For this review, take the finished solid that the model builds, in its own axes (mm). Round coordinates to 2 decimals unless told otherwise and drop trailing zeros. Order: outer loops, then holes, each group sorted by start corner. A loop starts at its lowest first (then second) coordinate and runs counter-clockwise, first axis right, second up. Notation, with made-up numbers: M 29.5,50.25 L 73.5,50.25 A5 ccw 73.5,56.25 Z; hole C 18,-35 d4. An arc over 180 degrees is marked long. Answer in a Markdown table with one row per item. Add a question column.
```python
from build123d import *

# Parameters (mm, degrees)
CYLINDER220_R     = 1.5
CYLINDER220_DEPTH = 10
CYLINDER093_R     = 4.1
CYLINDER093_DEPTH = 6.6


with BuildPart() as cylinder220:
    # Cylinder220 → Cylinder220 (new body)
    with BuildSketch(Plane.XY.offset(-1.9)):
        Circle(CYLINDER220_R)
    extrude(amount=CYLINDER220_DEPTH)


with BuildPart() as cut006:
    # Cylinder093 → Cylinder093 (new body)
    with BuildSketch(Plane.XY):
        Circle(CYLINDER093_R)
    extrude(amount=CYLINDER093_DEPTH)

    # Cut006: cut Cylinder220
    add(cylinder220.part, mode=Mode.SUBTRACT)


with BuildPart() as cut006_1:
    # Cut006 placement: moved
    add(cut006.part.moved(Location((76.8, 197.2, 52.1))))


solid = cut006_1.part
```
1. Consider section A-A on x = 76.8. Write out the cut boundary in (y, z), plus the area to 3 significant figures.
2. Clearance check with a flat-ended pin moving along its axis: pin 1 Ø1.5 at (y, z) = (198.5, 55.5) entering from -X. State where the tip first meets the part, or that it passes through.
3. Consider section D-D on x = 74.5. Write out the cut boundary in (y, z), plus the area to 3 significant figures.
4. The part is to be moulded in two halves that separate along Y. For faces 1 (the flat face through (77, 195, 52.1)), 2 (the cylindrical face through (78.69, 193.56, 55.35)), 3 (the cylindrical face through (76.475, 195.736, 55.354)), say which applies: pulls with the +Y half, pulls with the -Y half, needs draft (parallel to the pull), parting line crosses it, or undercut.
5. To check wall thickness, follow probe 1 along Y at (x, z) = (76.8, 55.5); probe 2 along X at (y, z) = (197.75, 56.75); probe 3 along X at (y, z) = (197, 54.25). State the ranges of each line that lie inside material, in increasing order. Write a range as [from, to].
6. Consider section B-B on y = 197.2. Write out the cut boundary in (x, z), plus the area to 3 significant figures.
7. Consider section C-C on z = 55. Write out the cut boundary in (x, y), plus the area to 3 significant figures.
Solved:
| question | item | result |
|---|---|---|
| 1 | outline | M 193.1,52.1 L 195.7,52.1 L 195.7,58.7 L 193.1,58.7 Z; M 198.7,52.1 L 201.3,52.1 L 201.3,58.7 L 198.7,58.7 Z |
| 1 | area | 34.3 mm^2 |
| 2 | pin 1 | stops at x = 72.74 |
| 3 | outline | M 193.81,52.1 L 200.59,52.1 L 200.59,58.7 L 193.81,58.7 Z |
| 3 | area | 44.8 mm^2 |
| 4 | face 1 | needs draft |
| 4 | face 2 | parting line crosses it |
| 4 | face 3 | undercut |
| 5 | probe 1 | y = [193.1, 195.7], [198.7, 201.3] |
| 5 | probe 2 | x = [72.74, 75.4], [78.2, 80.86] |
| 5 | probe 3 | x = [72.7, 75.31], [78.29, 80.9] |
| 6 | outline | M 72.7,52.1 L 75.3,52.1 L 75.3,58.7 L 72.7,58.7 Z; M 78.3,52.1 L 80.9,52.1 L 80.9,58.7 L 78.3,58.7 Z |
| 6 | area | 34.3 mm^2 |
| 7 | outline | C 76.8,197.2 d8.2; hole C 76.8,197.2 d3 |
| 7 | area | 45.7 mm^2 |
